from build123d import *

# Parameters (mm, degrees)
SKETCH1_W           = 77
SKETCH1_H           = 77
BOSS_EXTRUDE1_DEPTH = 2
SKETCH3_R           = 3.5
BOSS_EXTRUDE2_DEPTH = 4
SKETCH5_R           = 1.5
CUT_EXTRUDE1_DEPTH  = 57.341917038
CUT_EXTRUDE3_DEPTH  = 5
CIRPATTERN3_COUNT   = 4
FILLET3_R           = 4
CUT_EXTRUDE5_DEPTH  = 5
SKETCH6_R           = 1.5
CUT_EXTRUDE6_DEPTH  = 57.341917038
FILLET4_R           = 10
SKETCH8_R           = 5
CUT_EXTRUDE7_DEPTH  = 10
FILLET5_R           = 2


with BuildPart() as part:
    # Sketch1 → Boss-Extrude1 (new body)
    with BuildSketch(Plane(origin=(0, 0, 0), x_dir=(1, 0, 0), z_dir=(0, 1, 0))):
        Rectangle(SKETCH1_W, SKETCH1_H)
        Polygon((14.142135624, 24.748737342), (24.748737342, 14.142135624), (35.355339059, 24.748737342), (24.748737342, 35.355339059), align=None, mode=Mode.SUBTRACT)
        Polygon((-24.748737342, 14.142135624), (-35.355339059, 24.748737342), (-24.748737342, 35.355339059), (-14.142135624, 24.748737342), align=None, mode=Mode.SUBTRACT)
        Polygon((-14.142135624, -24.748737342), (-24.748737342, -14.142135624), (-35.355339059, -24.748737342), (-24.748737342, -35.355339059), align=None, mode=Mode.SUBTRACT)
        Polygon((14.142135624, -24.748737342), (24.748737342, -14.142135624), (35.355339059, -24.748737342), (24.748737342, -35.355339059), align=None, mode=Mode.SUBTRACT)
    extrude(amount=BOSS_EXTRUDE1_DEPTH)

    # Sketch3 → Boss-Extrude2 (add)
    with BuildSketch(Plane(origin=(0, 0, 0), x_dir=(1, 0, 0), z_dir=(0, 1, 0))):
        with Locations(Location((-36.239222536, 36.239222536, 0), (0, 0, 40.235921257))):
            Circle(SKETCH3_R)
        with Locations(Location((36.239222536, 36.239222536, 0), (0, 0, 139.764078743))):
            Circle(SKETCH3_R)
        with Locations(Location((-36.239222536, -36.239222536, 0), (0, 0, 130.235921257))):
            Circle(SKETCH3_R)
        with Locations(Location((36.239222536, -36.239222536, 0), (0, 0, 49.764078743))):
            Circle(SKETCH3_R)
    extrude(amount=BOSS_EXTRUDE2_DEPTH)

    # Sketch5 → Cut-Extrude1 (cut, through all)
    with BuildSketch(Plane(origin=(0, 0, 0), x_dir=(1, 0, 0), z_dir=(0, 1, 0))):
        with Locations(Location((0, 0, 0), (0, 0, 270))):
            Circle(SKETCH5_R)
    extrude(amount=CUT_EXTRUDE1_DEPTH, mode=Mode.SUBTRACT)

    # Sketch4 → Cut-Extrude3 (cut)
    with BuildSketch(Plane(origin=(0, 0, 0), x_dir=(1, 0, 0), z_dir=(0, 1, 0))):
        Polygon((-38.5, 23.5), (-38.5, -23.5), (-35.5, -20.5), (-35.5, 20.5), align=None)
    cut_extrude3 = extrude(amount=CUT_EXTRUDE3_DEPTH, mode=Mode.SUBTRACT)

    # CirPattern3: Cut-Extrude3 ×4 about axis
    cirpattern3_axis = Axis((0, 0, 0), (0, 1, 0))
    for i in range(1, CIRPATTERN3_COUNT):
        add(cut_extrude3.rotate(cirpattern3_axis, i * 360 / CIRPATTERN3_COUNT), mode=Mode.SUBTRACT)

    # Fillet3
    fillet3_edges = [part.edges().sort_by_distance(p)[0] for p in [
        (-38.5, 1, -23.5),
        (-38.5, 1, 23.5),
        (-35.5, 1, 20.5),
        (-23.5, 1, -38.5),
        (23.5, 1, -38.5),
        (-20.5, 1, -35.5),
        (38.5, 1, -23.5),
        (38.5, 1, 23.5),
        (35.5, 1, -20.5),
        (23.5, 1, 38.5),
        (-23.5, 1, 38.5),
        (20.5, 1, 35.5),
    ]]
    fillet(fillet3_edges, radius=FILLET3_R)

    # Sketch2 → Cut-Extrude5 (cut)
    with BuildSketch(Plane(origin=(0, 0, 0), x_dir=(1, 0, 0), z_dir=(0, 1, 0))):
        Polygon((35.355339059, 0), (0, 35.355339059), (-35.355339059, 0), (0, -35.355339059), align=None)
    extrude(amount=CUT_EXTRUDE5_DEPTH, mode=Mode.SUBTRACT)

    # Sketch6 → Cut-Extrude6 (cut, through all)
    with BuildSketch(Plane(origin=(0, 0, 0), x_dir=(1, 0, 0), z_dir=(0, 1, 0))):
        with Locations(Location((-36.239222536, 36.239222536, 0), (0, 0, 270))):
            Circle(SKETCH6_R)
        with Locations(Location((-36.239222536, -36.239222536, 0), (0, 0, 270))):
            Circle(SKETCH6_R)
        with Locations(Location((36.239222536, -36.239222536, 0), (0, 0, 270))):
            Circle(SKETCH6_R)
        with Locations(Location((36.239222536, 36.239222536, 0), (0, 0, 270))):
            Circle(SKETCH6_R)
    extrude(amount=CUT_EXTRUDE6_DEPTH, mode=Mode.SUBTRACT)

    # Fillet4
    fillet4_edges = [part.edges().sort_by_distance(p)[0] for p in [
        (0, 1, 35.355339059),
        (35.355339059, 1, 0),
        (0, 1, -35.355339059),
        (-35.355339059, 1, 0),
    ]]
    fillet(fillet4_edges, radius=FILLET4_R)

    # Sketch8 → Cut-Extrude7 (cut)
    with BuildSketch(Plane(origin=(0, 2, 0), x_dir=(1, 0, 0), z_dir=(0, 1, 0))):
        with Locations((15.556349186, 15.556349186)):
            Circle(SKETCH8_R)
        with Locations((-15.556349186, 15.556349186)):
            Circle(SKETCH8_R)
        with Locations((-15.556349186, -15.556349186)):
            Circle(SKETCH8_R)
        with Locations((15.556349186, -15.556349186)):
            Circle(SKETCH8_R)
    extrude(amount=-CUT_EXTRUDE7_DEPTH, mode=Mode.SUBTRACT)

    # Fillet5
    fillet5_edges = [part.edges().sort_by_distance(p)[0] for p in [
        (-24.395183951, 2, 10.960155108),
        (-24.395183951, 2, -10.960155108),
        (10.960155108, 2, 24.395183951),
        (-10.960155108, 2, 24.395183951),
        (24.395183951, 2, -10.960155108),
        (24.395183951, 2, 10.960155108),
        (-10.960155108, 2, -24.395183951),
        (10.960155108, 2, -24.395183951),
        (-31.213203436, 2, 0),
        (0, 2, 31.213203436),
        (31.213203436, 2, 0),
        (0, 2, -31.213203436),
    ]]
    fillet(fillet5_edges, radius=FILLET5_R - 0.0001)  # a hair under: the kernel refuses the full size


solid = part.part
For this review, take the finished solid that the model builds, in its own axes (mm). A direction names the side the tool comes from. Round coordinates to 2 decimals unless told otherwise and drop trailing zeros. Order: outer loops, then holes, each group sorted by start corner. A loop starts at its lowest first (then second) coordinate and runs counter-clockwise, first axis right, second up. Notation, with made-up numbers: (40.5, 10.25) -> (82.5, 10.25) arc R8 ccw to (82.5, 24.25) -> close; hole circle Ø10 at (47, 89). An arc over 180 degrees is marked (long way). Put each result on its own line as item: value.
Q1. Mouldability with a two-part tool opening along Z and no side actions: class faces 6 (the cylindrical face through (-20.39, 1.01, -35.81)), 7 (the flat face through (-35, 4, -35)), 8 (the cylindrical face through (-38.204, 1.014, 23.646)) as pulls with the +Z half, pulls with the -Z half, needs draft (parallel to the pull), parting line crosses it, or undercut.
Check result:
face 6: pulls with the -Z half
face 7: needs draft
face 8: undercut
Q2. Add section A-A on y = 2.85. Write out the cut boundary in (x, z).
Check result:
outline: circle Ø7 at (-36.24, -36.24); circle Ø7 at (-36.24, 36.24); circle Ø7 at (36.24, -36.24); circle Ø7 at (36.24, 36.24); hole circle Ø3 at (-36.24, -36.24); hole circle Ø3 at (-36.24, 36.24); hole circle Ø3 at (36.24, -36.24); hole circle Ø3 at (36.24, 36.24)
Q3. Machinability: for faces 1 (the cylindrical face through (-24.67, 1.43, 11.54)), 2 (the flat face through (-29, 1, 38.5)), 3 (the flat face through (19.37, 0.99, -19.52)), 4 (the flat face through (35.5, 1, 1)), 5 (the cylindrical face through (23.61, 1.01, -38.19)), which of the approach directions +Z, -Z, +X, -X, +Y, -Y give a long, thin tool a straight path to every point of the face, cutting with its end or side? Answer none if there is none.
Check result:
face 1: +Y
face 2: +Z, +Y, -Y
face 3: +Y, -Y
face 4: +X, +Y, -Y
face 5: -Z, +Y, -Y
Q4. For probe 1 along Z at (x, y) = (-18, 0.5); probe 2 along X at (y, z) = (0.45, 34); probe 3 along Y at (x, z) = (11.5, -31), list the stretches that pass through material, from the lowest coordinate up. Write a range as [from, to].
Check result:
probe 1: [-35.5, -28.61], [-20.89, -19.92], [19.92, 20.89], [28.61, 35.5]
probe 2: [-38.93, -26.1], [-23.39, 23.39], [26.1, 38.93]
probe 3: [0, 2]
Q5. Insertion check: pin 1 Ø1 at (y, z) = (1, -29.5) entering from +X; pin 2 Ø1.6 at (y, z) = (0.5, 27.5) entering from -X; pin 3 Ø2 at (y, z) = (1, -7.5) entering from -X. Each pin has a flat end and moves straight along its axis. Give the tip position at first contact, or say it passes through.
Check result:
pin 1: x = 38.5
pin 2: x = -38.5
pin 3: x = -35.5
